The listing builds one solid part. Answer for the finished solid, in the listing's coordinates (mm). A direction names the side the tool comes from. Round coordinates to 2 decimals unless told otherwise and drop trailing zeros. Write each loop counter-clockwise with the first axis right and the second up, starting at its lowest first coordinate (ties: lowest second). Pieces come first, ordered by that corner, then holes.
Item 1: Each of these flat-tipped pins is pushed along its axis until it touches: pin 1 (12 mm diameter, centred on x = 178, z = 9, fed in from -Y); pin 2 (4 mm diameter, centred on y = 39.5, z = 18.5, fed in from +X); pin 3 (2 mm diameter, centred on x = 45.5, z = 6, fed in from +Y). Where does it stop, or does it pass through?
Item 2: Find the intervals of material crossed by probe 1 along Y at (x, z) = (168.5, 24.75); probe 2 along X at (y, z) = (47, 26.25); probe 3 along Y at (x, z) = (31, 13.5), in increasing order.
Item 3: Find section A-A on y = 53.5. Give the vertices of the cut face in (x, z).
Item 4: For a pull along Y with two mould halves and no side action, classify faces 4 (the face through (165, 80, 20)), 5 (the face through (40, 91, 25)), 6 (the face through (170, 93, 28)) as +Y half, -Y half, draft (parallel to the pull), parting line (faces both ways), or undercut.
Item 5: Find section B-B on x = 57. Give the vertices of the cut face in (y, z), then the cut area to 3 significant figures.
Item 6: A tool of negligible diameter and unlimited length cuts with its end or side. For faces 1 (the face through (15, 87, 10)), 2 (the face through (109.619, 83.521, 21.915)), 3 (the face through (165, 10, 20)), from which of +Z, -Z, +X, -X, +Y, -Y can it reach the whole face along a straight path? Write none if from no direction.
Item 7: Find section C-C on y = 65. Give the vertices of the cut face in (x, z), then the cut area to 3 significant figures.
Autodesk Fusion 360 part; units mm, degrees
sketch "Sketch1" plane through (0, 0, 0) normal (0, 0, 1) x (1, 0, 0)
  line L0 (0, 90) -> (210, 90)
  line L1 (210, 90) -> (210, 0)
  line L2 (210, 0) -> (0, 0)
  line L3 (0, 0) -> (0, 90)
  line L4 (5, 5) -> (205, 5)
  line L5 (205, 5) -> (205, 85)
  line L6 (205, 85) -> (5, 85)
  line L7 (5, 85) -> (5, 5)
  dimension "d1" = 210
  dimension "d2" = 90
  dimension "d3" = 200
  dimension "d4" = 80
  dimension "d5" = 5
  dimension "d6" = 5
extrude "Extrude1" add sketch "Sketch1" along normal blind 5 contours L4 L5 L6 L7
extrude "Extrude2" add sketch "Sketch1" along normal blind 30
sketch "Sketch3" plane through (0, 85, 0) normal (0, -1, 0) x (1, 0, 0)
  line L0 (5, 5) -> (205, 5)
  line L1 (205, 5) -> (205, 30)
  line L2 (205, 30) -> (5, 30)
  line L3 (5, 30) -> (5, 5)
  circle A0 centre (105, 20) radius 5
  line L4 (210, 0) -> (210, 30)
  circle A1 centre (165, 20) radius 5
  dimension "d15" = 10
  dimension "d16" = 10
  dimension "d17" = 105
  dimension "d80" = 10
  dimension "d81" = 60
extrude "Extrude3" add sketch "Sketch3" along normal blind 5 contours A0
sketch "Sketch4" plane through (0, 80, 0) normal (0, -1, 0) x (1, 0, 0)
  circle A0 centre (105, 20) radius 5
  circle A1 centre (105, 20) radius 7.5
  dimension "d20" = 15
extrude "Extrude4" add sketch "Sketch4" against normal blind 2
sketch "Sketch6" plane through (0, 85, 0) normal (0, -1, 0) x (1, 0, 0)
  circle A0 centre (105, 20) radius 5
  line L0 (5, 5) -> (205, 5)
  line L1 (205, 5) -> (205, 30)
  line L2 (205, 30) -> (5, 30)
  line L3 (5, 30) -> (5, 5)
  line L4 (162, 11) -> (168, 11)
  line L5 (168, 11) -> (168, 5)
  line L6 (168, 5) -> (162, 5)
  line L7 (162, 5) -> (162, 11)
  line L8 (5, 5) -> (205, 5)
  line L9 (210, 0) -> (210, 30)
  line L10 (162, 11) -> (168, 11)
  line L11 (168, 11) -> (168, 13)
  line L12 (168, 13) -> (162, 13)
  line L13 (162, 13) -> (162, 11)
  line L14 (168, 9) -> (170, 9)
  line L15 (170, 9) -> (170, 7)
  line L16 (170, 7) -> (168, 7)
  line L17 (168, 7) -> (168, 9)
  line L18 (162, 9) -> (160, 9)
  line L19 (160, 9) -> (160, 7)
  line L20 (160, 7) -> (162, 7)
  line L21 (162, 7) -> (162, 9)
  dimension "d91" = 6
  dimension "d92" = 6
  dimension "d93" = 42
  dimension "d94" = 2
  dimension "d95" = 2
  dimension "d96" = 2
  dimension "d97" = 2
  dimension "d98" = 2
  dimension "d99" = 2
  dimension "d100" = 2
sketch "Sketch7" plane through (0, 0, 0) normal (-1, 0, 0) x (0, -1, 0)
  line L0 (-90, 0) -> (0, 0)
  line L1 (0, 0) -> (0, 30)
  line L2 (0, 30) -> (-90, 30)
  line L3 (-90, 30) -> (-90, 0)
  circle A0 centre (-25, 30) radius 5
  line L4 (-30, 30) -> (-20, 30)
  circle A1 centre (-65, 30) radius 5
  line L5 (-70, 30) -> (-60, 30)
  dimension "d31" = 10
  dimension "d32" = 10
  dimension "d47" = 25
  dimension "d48" = 25
extrude "Extrude5" add sketch "Sketch7" along normal blind 3 contours L2 A1 L5 | L2 A0 L4 picked at (-66.5016, 29.2769) picked at (-23.5675, 28.3215)
ref_plane "WorkPlane1" through (0, 45, 0) normal (0, 1, 0) x (0, 0, 1)
mirror "Mirror1" about plane through (0, 45, 0) normal (0, 1, 0) of bodies 1 merged
ref_plane "WorkPlane2" through (105, 45, 15) normal (-1, 0, 0) x (0, -1, 0)
mirror "Mirror2" about plane through (105, 45, 15) normal (-1, 0, 0) of bodies 1 merged
sketch "Sketch8" plane through (0, 0, 0) normal (0, -1, 0) x (1, 0, 0)
  line L0 (0, 0) -> (210, 0)
  line L1 (210, 0) -> (210, 30)
  line L2 (210, 30) -> (0, 30)
  line L3 (0, 30) -> (0, 0)
  circle A0 centre (40, 30) radius 5
  circle A1 centre (170, 30) radius 5
  line L4 (35, 30) -> (45, 30)
  line L5 (165, 30) -> (175, 30)
  dimension "d39" = 10
  dimension "d40" = 10
  dimension "d41" = 40
  dimension "d42" = 40
extrude "Extrude6" add sketch "Sketch8" along normal blind 3 contours L2 A0 L4 | L2 A1 L5 picked at (38.7453, 27.2668) picked at (169.3911, 27.9517)
mirror "Mirror3" about plane through (0, 45, 0) normal (0, 1, 0) of bodies 1 merged
sketch "Sketch9" plane through (105, 85, 17.5) normal (0, -1, 0) x (1, 0, 0)
  line L0 (-100, -12.5) -> (-90, -12.5)
  line L1 (-90, -12.5) -> (-90, -2.5)
  line L2 (-90, -2.5) -> (-100, -2.5)
  line L3 (-100, -2.5) -> (-100, -12.5)
  line L4 (105, -17.5) -> (-105, -17.5)
  point P0 (-105, -17.5)
  dimension "d49" = 10
  dimension "d50" = 10
  dimension "d51" = 5
  dimension "d52" = 5
sketch "Sketch10" plane through (0, 0, 5) normal (0, 0, 1) x (-1, 0, 0)
  line L0 (-5, -85) -> (-5, -5)
  line L1 (-5, -5) -> (-205, -5)
  line L2 (-205, -5) -> (-205, -85)
  line L3 (-205, -85) -> (-5, -85)
  circle A0 centre (-45, -45) radius 20
  circle A1 centre (-105, -45) radius 20
  circle A2 centre (-165, -45) radius 20
  line L4 (-210, -90) -> (-210, 0)
  line L5 (-210, 0) -> (0, 0)
  line L6 (-42, -48) -> (-48, -48)
  line L7 (-48, -48) -> (-48, -42)
  line L8 (-48, -42) -> (-42, -42)
  line L9 (-42, -42) -> (-42, -48)
  line L10 (-48, -48) -> (-50, -48)
  line L11 (-50, -48) -> (-50, -42)
  line L12 (-50, -42) -> (-48, -42)
  line L13 (-48, -42) -> (-48, -48)
  line L14 (-42, -48) -> (-40, -48)
  line L15 (-40, -48) -> (-40, -42)
  line L16 (-40, -42) -> (-42, -42)
  line L17 (-42, -42) -> (-42, -48)
  line L18 (-44, -50) -> (-46, -50)
  line L19 (-46, -50) -> (-46, -48)
  line L20 (-46, -48) -> (-44, -48)
  line L21 (-44, -48) -> (-44, -50)
  line L22 (-44, -42) -> (-46, -42)
  line L23 (-46, -42) -> (-46, -40)
  line L24 (-46, -40) -> (-44, -40)
  line L25 (-44, -40) -> (-44, -42)
  dimension "d55" = 40
  dimension "d56" = 40
  dimension "d57" = 40
  dimension "d58" = 105
  dimension "d59" = 60
  dimension "d60" = 60
  dimension "d61" = 45
  dimension "d62" = 45
  dimension "d63" = 45
  dimension "d64" = 6
  dimension "d65" = 6
  dimension "d66" = 3
  dimension "d67" = 3
  dimension "d68" = 2
  dimension "d69" = 2
  dimension "d70" = 2
  dimension "d71" = 2
  dimension "d72" = 2
  dimension "d73" = 2
  dimension "d74" = 2
  dimension "d75" = 2
  dimension "d76" = 6
extrude "Extrude8" add sketch "Sketch10" along normal blind 2 contours L9 L14 L15 L16 L17 | L6 L18 L19 L20 L21 | L8 L22 L23 L24 L25 | L7 L10 L11 L12 L13
extrude "Extrude9" add sketch "Sketch3" along normal blind 5 contours A1
sketch "Sketch11" plane through (0, 80, 0) normal (0, -1, 0) x (1, 0, 0)
  circle A0 centre (165, 20) radius 5
  circle A1 centre (165, 20) radius 7.5
  dimension "d84" = 15
extrude "Extrude10" add sketch "Sketch11" against normal blind 2
mirror "Mirror4" about plane through (0, 45, 0) normal (0, 1, 0) of bodies 1 merged
extrude "Extrude11" cut sketch "Sketch9" against normal blind 5
extrude "Extrude12" add sketch "Sketch6" along normal blind 2 contours L7 L18 L19 L20 L21 | L5 L14 L15 L16 L17 | L4 L10 L11 L12 L13
Check values:
1. pin 1: stops at y = 0
1. pin 2: stops at x = 210
1. pin 3: stops at y = 90
2. probe 1: y = 0 to 5, 8 to 10, 80 to 82, 85 to 90
2. probe 2: x = 0 to 5, 205 to 210
2. probe 3: y = 0 to 5, 85 to 90
3. outline: (0, 0) - (210, 0) - (210, 30) - (205, 30) - (205, 5) - (5, 5) - (5, 30) - (0, 30) - close
4. face 4: undercut
4. face 5: draft
4. face 6: +Y half
5. outline: (0, 0) - (90, 0) - (90, 30) - (85, 30) - (85, 5) - (5, 5) - (5, 30) - (0, 30) - close
5. area: 700 mm2
6. face 1: +Y
6. face 2: none
6. face 3: +Z
7. outline: (-3, 25) - (0, 25) - (0, 0) - (210, 0) - (210, 25) - (213, 25) - (213, 30) - (205, 30) - (205, 5) - (5, 5) - (5, 30) - (-3, 30) - close
7. area: 1,330 mm2
